Autodesk Inventor part; units mm, degrees
ref_plane "YZ Plane" through (0, 0, 0) normal (1, 0, 0) x (0, 1, 0)
ref_plane "XZ Plane" through (0, 0, 0) normal (0, 1, 0) x (-1, 0, 0)
ref_plane "XY Plane" through (0, 0, 0) normal (0, 0, 1) x (1, 0, 0)
sketch "Sketch1" plane through (0, 0, 0) normal (1, 0, 0) x (0, 1, 0)
  line L0 (67.2039, 7.058) -> (87.2039, 7.058)
  line L1 (87.2039, 7.058) -> (87.2039, 31.058)
  line L2 (87.2039, 31.058) -> (-82.7961, 31.058)
  line L3 (-82.7961, 31.058) -> (-82.7961, 24.058)
  line L4 (-82.7961, 24.058) -> (80.2039, 24.058)
  line L5 (80.2039, 24.058) -> (80.2039, 14.058)
  line L6 (80.2039, 14.058) -> (67.2039, 14.058)
  line L7 (67.2039, 14.058) -> (67.2039, 7.058)
  dimension "d0" = 10
  dimension "d1" = 13
  dimension "d2" = 7
  dimension "d3" = 7
  dimension "d5" = 7
  dimension "d6" = 170
extrude "Extrusion1" add sketch "Sketch1" along normal blind 15
sketch "Sketch2" plane through (15, 0, 0) normal (1, 0, 0) x (0, 0, -1)
  line L0 (-7.058, 67.2039) -> (-7.058, 87.2039)
  line L1 (-7.058, 87.2039) -> (-31.058, 87.2039)
  line L2 (-31.058, 87.2039) -> (-31.058, -82.7961)
  line L3 (-31.058, -82.7961) -> (-24.058, -82.7961)
  line L4 (-24.058, -82.7961) -> (-24.058, 80.2039)
  line L5 (-24.058, 80.2039) -> (-14.058, 80.2039)
  line L6 (-14.058, 80.2039) -> (-14.058, 67.2039)
  line L7 (-14.058, 67.2039) -> (-7.058, 67.2039)
  line L8 (-31.058, 52.2039) -> (-24.058, 52.2039)
  line L9 (-24.058, 80.2039) -> (-24.058, -82.7961)
  line L10 (-24.058, 67.2039) -> (-31.058, 67.2039)
  point P0 (0, 0)
  dimension "d9" = 15
  dimension "d10" = 20
extrude "Extrusion2" add sketch "Sketch2" along normal blind 135 contours L10 L4 L8 L2
fillet "Fillet1" radius 5 2 edges at (15, 67.2039, 27.558) (15, 52.2039, 27.558)
ref_plane "Work Plane1" through (0, 67.2039, 10.558) normal (0, 0, 1) x (1, 0, 0)
sketch "Sketch6" plane through (150, 0, 0) normal (1, 0, 0) x (0, 0, -1)
  line L0 (-31.058, 52.2039) -> (-24.058, 52.2039)
  line L1 (-24.058, 52.2039) -> (-24.058, 67.2039)
  line L2 (-24.058, 67.2039) -> (-31.058, 67.2039)
  line L3 (-31.058, 67.2039) -> (-31.058, 52.2039)
  line L4 (-31.058, 54.4039) -> (-29.058, 54.4039)
  line L5 (-29.058, 54.4039) -> (-29.058, 65.0039)
  line L6 (-29.058, 65.0039) -> (-31.058, 65.0039)
  line L7 (-31.058, 67.2039) -> (-31.058, 52.2039) construction
  line L8 (-31.058, 59.7039) -> (-29.058, 59.7039) construction
  point P0 (0, 0)
  dimension "d23" = 10.6
  dimension "d24" = 2
sketch "Sketch7" plane through (0, -82.7961, 31.058) normal (0, 0, 1) x (1, 0, 0)
  line L0 (0, 0) -> (0, 170)
  line L1 (0, 0) -> (15, 0)
  line L2 (15, 130) -> (15, 0)
  arc A0 (20, 135) -> (15, 130) centre (20, 130) ccw
  line L3 (20, 135) -> (150, 135)
  line L4 (150, 150) -> (150, 135)
  line L5 (20, 150) -> (150, 150)
  arc A1 (15, 155) -> (20, 150) centre (20, 155) ccw
  line L6 (15, 170) -> (15, 155)
  line L7 (0, 170) -> (15, 170)
  arc A2 (20, 142.5) -> (7.5, 130) centre (20, 130) ccw
  line L8 (150, 135) -> (150, 150)
  line L9 (150, 142.5) -> (20, 142.5)
  line L10 (0, 0) -> (15, 0)
  line L11 (7.5, 0) -> (7.5, 130)
  point P0 (0, 82.7961)
  dimension "d25" = 7.5
sweep "Sweep1" cut profiles "Sketch6" path "Sketch7" path curves L9 A2 L11 contours L3 L6 L5 L4
sketch "Sketch8" plane through (0, -82.7961, 31.058) normal (0, 0, 1) x (1, 0, 0)
  line L0 (150, 147.8) -> (150, 137.2)
  line L1 (150, 147.8) -> (20, 147.8)
  arc A0 (20, 147.8) -> (2.2, 130) centre (20, 130) ccw
  line L2 (2.2, 130) -> (2.2, 0)
  line L3 (12.8, 0) -> (2.2, 0)
  line L4 (12.8, 130) -> (12.8, 0)
  arc A1 (20, 137.2) -> (12.8, 130) centre (20, 130) ccw
  line L5 (150, 137.2) -> (20, 137.2)
  line L6 (2.2, 0) -> (2.2, 130)
  arc A2 (20, 147.8) -> (2.2, 130) centre (20, 130) ccw
  line L7 (20, 147.8) -> (150, 147.8)
  line L8 (150, 150) -> (150, 147.8)
  line L9 (20, 150) -> (150, 150)
  arc A3 (15, 155) -> (20, 150) centre (20, 155) ccw
  line L10 (15, 170) -> (15, 155)
  line L11 (0, 170) -> (15, 170)
  line L12 (0, 0) -> (0, 170)
  line L13 (0, 0) -> (2.2, 0)
  line L14 (12.8, 130) -> (12.8, 0)
  line L15 (12.8, 0) -> (15, 0)
  line L16 (15, 130) -> (15, 0)
  arc A4 (20, 135) -> (15, 130) centre (20, 130) ccw
  line L17 (20, 135) -> (150, 135)
  line L18 (150, 137.2) -> (150, 135)
  line L19 (150, 137.2) -> (20, 137.2)
  arc A5 (20, 137.2) -> (12.8, 130) centre (20, 130) ccw
  line L20 (150, 135) -> (150, 150)
  line L21 (150, 142.5) -> (135.884, 142.5) construction
  line L22 (150, 145) -> (140, 147.8)
  line L23 (150, 147.8) -> (20, 147.8) construction
  line L24 (140, 147.8) -> (135, 147.8)
  line L25 (135, 147.8) -> (135, 137.2)
  line L26 (150, 137.2) -> (20, 137.2)
  line L27 (135, 137.2) -> (140, 137.2)
  line L28 (150, 140) -> (140, 137.2)
  line L29 (150, 140) -> (150, 145) construction
  line L30 (150, 145) -> (150, 140)
  point P0 (0, 82.7961)
  dimension "d29" = 5
  dimension "d30" = 5
  dimension "d31" = 15
  dimension "d32" = 5
extrude "Extrusion5" cut sketch "Sketch8" against normal blind 5.75 contours L0 L28 L5 L25 L1 L22
fillet "Fillet2" radius 4 2 edges at (7.5, 87.2039, 31.058) (7.5, 87.2039, 7.058)
fillet "Fillet3" radius 2 2 edges at (7.5, 80.2039, 24.058) (7.5, 80.2039, 14.058)
fillet "Fillet4" radius 2 2 edges at (7.5, 67.2039, 7.058) (7.5, 67.2039, 14.058)
sketch "Sketch9" plane through (20, 67.2039, 31.058) normal (0, 0, 1) x (1, 0, 0)
  line L0 (-20, 16) -> (-5, 16)
  line L1 (-5, 16) -> (-5, 5)
  circle A0 centre (-12.5, 9.6858) radius 2.175
  line L2 (-12.5, 16) -> (-12.5, 9.6858) construction
  line L3 (-5, 9.6858) -> (-12.5, 9.6858) construction
  point P0 (-20, -67.2039)
  dimension "d38" = 4.35
  dimension "d39" = 6.3142
extrude "Extrusion6" cut sketch "Sketch9" against normal blind 10
ref_plane "Work Plane2" through (20, 67.2039, 27.558) normal (0, 0, 1) x (1, 0, 0)
sketch "Sketch10" plane through (20, 67.2039, 27.558) normal (0, 0, 1) x (1, 0, 0)
  line L0 (-14.2331, 11) -> (-20, 11)
  line L1 (-20, 11) -> (-20, 13)
  line L2 (-20, 13) -> (-5, 13)
  line L3 (-5, 13) -> (-5, 11)
  line L4 (-5, 11) -> (-10.7669, 11)
  arc A0 (-14.2331, 11) -> (-10.7669, 11) centre (-12.5, 9.6858) ccw
  line L5 (-5, 11) -> (-10.7669, 11)
  line L6 (-5, 5) -> (-5, 11)
  arc A1 (-5, 5) -> (0, 0) centre (0, 5) ccw
  line L7 (0, 0) -> (130, 0)
  line L8 (130, -15) -> (130, 0)
  line L9 (130, -15) -> (0, -15)
  arc A2 (0, -15) -> (-5, -20) centre (0, -20) ccw
  line L10 (-5, -150) -> (-5, -20)
  line L11 (-20, -150) -> (-5, -150)
  line L12 (-20, 11) -> (-20, -150)
  line L13 (-14.2331, 11) -> (-20, 11)
  line L14 (-10.4071, 6.0608) -> (-14.5929, 6.0608)
  line L15 (-14.5929, 6.0608) -> (-16.6858, 9.6858)
  line L16 (-16.6858, 9.6858) -> (-14.5929, 13.3108)
  line L17 (-14.5929, 13.3108) -> (-10.4071, 13.3108)
  line L18 (-8.3142, 9.6858) -> (-12.5, 9.6858) construction
  line L19 (-10.4071, 13.3108) -> (-5, 13.3108)
  line L20 (-5, 2) -> (-5, 16)
  line L21 (-10.4071, 6.0608) -> (-5, 6.0608)
  line L22 (-5, 6.0608) -> (-5, 13.3108)
  line L23 (-10.4071, 13.3108) -> (-10.372, 13)
  point P0 (-20, -67.2039)
  dimension "d42" = 7.25
extrude "Extrusion7" cut sketch "Sketch10" along normal mid plane 4 contours A0 L4 L6 L21 L14 L15 L16 L0 | L0 L16 L2 L3 L4 A0 | L16 L17 L23 L2 | L23 L19 L20 L2
equation "\"d3\" = d2"
equation "\"d5\" = d2"
equation "\"d30\" = d29"
properties part number "Top Clip"
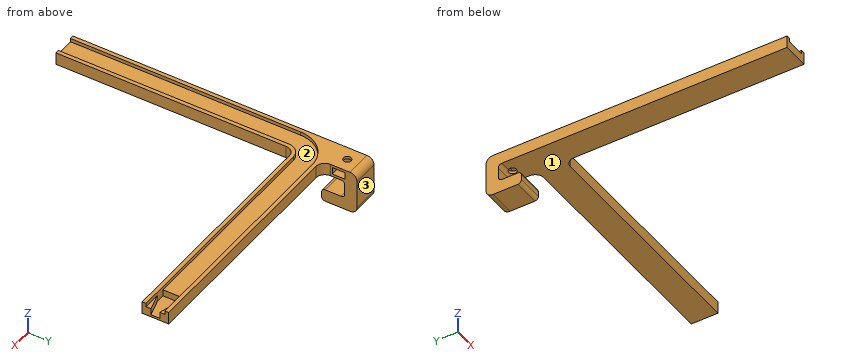
Model file for the job. Use its own axes, mm. Face numbers are marked on the shaded views. Give positions to 0.01 mm unless a question says otherwise; leave off trailing zeros. Write each loop counter-clockwise with the first axis right and the second up, starting at its lowest first coordinate (ties: lowest second). Pieces come first, ordered by that corner, then holes. Notation, with made-up numbers: (-19, -31) -> (1, -31) arc R17 cw to (1, -24) -> close; hole circle Ø11 at (6.25, -7). An arc over 180 degrees is marked (long way). Use CSV: the item, a comma, the result in double quotes. Start each with the question number.
1) Cut at A-A on x = 40. List the corners of the cut face in (y, z), plus the area to 3 significant figures.
2) Cut at B-B on y = 39. List the corners of the cut face in (x, z), plus the area to 3 significant figures.
3) Drill centre lines: L1, parallel to Y at x = 139, z = 26.5; L2, parallel to Y at x = 7.5, z = 24.6; L3, parallel to Z at x = 9, y = -30. Where is each one in solid material? Low to high.
4) Two-plate mould, pull along Y, no slides. Class the marked faces 1, 2 and 3: released by +Y, released by -Y, zero draft, split by the parting line, or undercut.
5) Pin check, flat tips, straight feed: P1, Ø10, axis at y = -25.5, z = 25.5, coming from the +X side; P2, Ø7.5, axis at x = 112.5, z = 28, coming from the -Y side; P3, Ø1.8, axis at x = 10, z = 18.5, coming from the -Y side. Stop position of each tip, or through.
Final values:
1,outline,"(52.2, 24.06) -> (67.2, 24.06) -> (67.2, 31.06) -> (65, 31.06) -> (65, 29.06) -> (54.4, 29.06) -> (54.4, 31.06) -> (52.2, 31.06) -> close"
1,area,"83.8 mm2"
2,outline,"(0, 24.06) -> (15, 24.06) -> (15, 31.06) -> (12.8, 31.06) -> (12.8, 29.06) -> (2.2, 29.06) -> (2.2, 31.06) -> (0, 31.06) -> close"
2,area,"83.8 mm2"
3,L1,"y = 52.2 to 54.4, 65 to 67.2"
3,L2,"y = -82.8 to 74.71, 79.06 to 87.2"
3,L3,"z = 24.06 to 29.06"
4,face 1,"zero draft"
4,face 2,"undercut"
4,face 3,"released by +Y"
5,P1,"stops at x = 15"
5,P2,"stops at y = 52.2"
5,P3,"stops at y = 80.2"
